```python
from build123d import *

# Parameters (mm, degrees)
SKETCH_1_W           = 0.75
SKETCH_1_H           = 20
EXTRUDE_2_DEPTH      = 0.25
EXTRUDE_2_DEPTH_BACK = 0.25
SKETCH_3_R           = 0.5


with BuildPart() as part:
    # Sketch 1 → Revolve 4 (revolve)
    with BuildSketch(Plane.XY, mode=Mode.PRIVATE) as revolve_4_sk:
        with Locations((1.875, 10)):
            Rectangle(SKETCH_1_W, SKETCH_1_H)
    revolve(revolve_4_sk.sketch.rotate(Axis((1.5, 20, 0), (0, -1, 0)), 90), axis=Axis((1.5, 20, 0), (0, -1, 0)))

    # Sketch 3 → Extrude 2 (add, two sides: drawn at the far end of the back side and taken through both)
    with BuildSketch(Plane.XY.offset(-EXTRUDE_2_DEPTH_BACK)):
        with BuildLine():
            Line((0.75, 0), (0.75, -0.75))
            ThreePointArc((0.75, -0.75), (1.5, -1.5), (2.25, -0.75))
            Line((2.25, -0.75), (2.25, 0))
            Line((2.25, 0), (0.75, 0))
        make_face()
        with Locations((1.5, -0.75)):
            Circle(SKETCH_3_R, mode=Mode.SUBTRACT)
    extrude(amount=EXTRUDE_2_DEPTH + EXTRUDE_2_DEPTH_BACK)


solid = part.part
```
Input: part model. Units: mm. Frame: model coordinates. Round coordinates to 2 decimals unless told otherwise and drop trailing zeros. Write each loop counter-clockwise with the first axis right and the second up, starting at its lowest first coordinate (ties: lowest second). Pieces come first, ordered by that corner, then holes. Notation, with made-up numbers: M 72,42 L 81,42 A16 cw 81,47 Z; hole C 68.5,-25.5 d3. An arc over 180 degrees is marked long. Write each question's results on one line, items separated by ' | '.
Q1. Section query C-C (z = 0.45). Return loops of the section in (x, y), and give its area (3 significant figures).
Results:
outline: M 0.9,0 L 2.1,0 L 2.1,20 L 0.9,20 Z | area: 24.0 mm^2
Q2. Draft query along X for faces 1 (the face through (1, 20, 0)), 2 (the face through (0.756, 10.14, -0.098)), 3 (the face through (1.1, -1.05, 0)). Return one class per face: released by +X, released by -X, zero draft, split by the parting line, or undercut.
Results:
face 1: zero draft | face 2: split by the parting line | face 3: undercut
Q3. Pin query (flat end, axial travel): P1, Ø0.8, axis at x = 1.5, y = -0.5, coming from the -Z side. Return the tip coordinate at first contact, or that it passes through.
Results:
P1: stops at z = -0.25
Q4. Line query: line 1 along Y through (x, z) = (1.45, 0); line 2 along Z through (x, y) = (1.45, 18.5); line 3 along X through (y, z) = (18.75, -0.05). Output: solid intervals per line, ascending.
Results:
line 1: y = -1.5 to -1.25, -0.25 to 20 | line 2: z = -0.75 to 0.75 | line 3: x = 0.75 to 2.25
Q5. Section query A-A (x = 1.5). Return loops of the section in (y, z), and give its area (4 significant figures).
Results:
outline: M -1.5,-0.25 L -1.25,-0.25 L -1.25,0.25 L -1.5,0.25 Z; M -0.25,-0.25 L 0,-0.25 L 0,-0.75 L 20,-0.75 L 20,0.75 L 0,0.75 L 0,0.25 L -0.25,0.25 Z | area: 30.25 mm^2
Q6. Section query B-B (y = 8.75). Return loops of the section in (x, z).
Results:
outline: C 1.5,0 d1.5
